Can you work these out from the model? Positions are in its coordinate system, mm. A direction names the side the tool comes from. Give positions to 0.01 mm unless a question says otherwise; leave off trailing zeros. Order: outer loops, then holes, each group sorted by start corner. A loop starts at its lowest first (then second) coordinate and runs counter-clockwise, first axis right, second up. Notation, with made-up numbers: (-4.5, 36) - (4.5, 36) arc R12 ccw to (4.5, 45) - close; hole circle Ø9 at (-12, 14.5). An arc over 180 degrees is marked (long way). Answer as a JSON object with one key per item and string values.
```python
from build123d import *

# Parameters (mm, degrees)
SKETCH1_W                                            = 160
SKETCH1_H                                            = 20
BOSS_EXTRUDE1_DEPTH                                  = 10
CBORE_FOR_M6_SLOTTED_CHEESE_HEAD_SCREWS2_D           = 6.6
CBORE_FOR_M6_SLOTTED_CHEESE_HEAD_SCREWS2_CBORE_D     = 11
CBORE_FOR_M6_SLOTTED_CHEESE_HEAD_SCREWS2_CBORE_DEPTH = 6.8
M6_TAPPED_HOLE1_D                                    = 5
M6_TAPPED_HOLE1_DEPTH                                = 15
M6_TAPPED_HOLE1_TIP                                  = 1.502151548
CHAMFER1_SIZE                                        = 5


with BuildPart() as part:
    # Sketch1 → Boss-Extrude1 (new, symmetric)
    with BuildSketch(Plane(origin=(0, 0, 0), x_dir=(1, 0, 0), z_dir=(0, 1, 0))):
        Rectangle(SKETCH1_W, SKETCH1_H)
    extrude(amount=BOSS_EXTRUDE1_DEPTH, both=True)

    # CBORE for M6 Slotted cheese head screws2 (through all)
    with Locations(Plane(origin=(0, 10, 0), x_dir=(1, 0, 0), z_dir=(0, 1, 0))):
        with Locations((-16.182, 0), (63.818, 0)):
            CounterBoreHole(CBORE_FOR_M6_SLOTTED_CHEESE_HEAD_SCREWS2_D / 2, CBORE_FOR_M6_SLOTTED_CHEESE_HEAD_SCREWS2_CBORE_D / 2, CBORE_FOR_M6_SLOTTED_CHEESE_HEAD_SCREWS2_CBORE_DEPTH)

    # M6 Tapped Hole1
    with Locations(Plane.ZY.offset(80)):
        with Locations((0, 0)):
            Hole(M6_TAPPED_HOLE1_D / 2, depth=M6_TAPPED_HOLE1_DEPTH)
            with Locations((0, 0, -(M6_TAPPED_HOLE1_DEPTH + M6_TAPPED_HOLE1_TIP / 2))):  # 118° drill point
                Cone(0, M6_TAPPED_HOLE1_D / 2, M6_TAPPED_HOLE1_TIP, mode=Mode.SUBTRACT)

    # Chamfer1
    chamfer1_edges = [part.edges().sort_by_distance(p)[0] for p in [
        (80, 10, 0),
    ]]
    chamfer(chamfer1_edges, length=CHAMFER1_SIZE)


solid = part.part
```
Q1. I'm going to push flat-ended pins straight in: pin 1 Ø6 at (x, z) = (-16.182, 0) entering from -Y; pin 2 Ø10.5 at (x, z) = (63.818, 0) entering from +Y. Where does each tip first touch, or does it pass through?
Recorded:
{"pin 1": "passes through", "pin 2": "stops at y = 3.2"}
Q2. I need wall thicknesses on L1, parallel to X at y = 9.25, z = 4.5; L2, parallel to X at y = 8.25, z = 4; L3, parallel to Y at x = -14.5, z = 4. Which ranges of each line are inside material? Lowest first, please.
Recorded:
{"L1": "x = -80 to -19.34, -13.02 to 60.66, 66.98 to 75.75", "L2": "x = -80 to -19.96, -12.41 to 60.04, 67.59 to 76.75", "L3": "y = -10 to 3.2"}
Q3. If we section it at A-A, the plane y = -6.5: Please give me the cut outline in (x, z), then the cut area to 3 significant figures.
Recorded:
{"outline": "(-80, -10) - (80, -10) - (80, 10) - (-80, 10) - close; hole circle Ø6.6 at (-16.18, 0); hole circle Ø6.6 at (63.82, 0)", "area": "3,130 mm^2"}
Q4. We'd pull the mould along X, two halves only. Please class faces 1 (the face through (64, 3.2, 4)), 2 (the face through (80, -2, 0)), 3 (the face through (-80, -2, 2)): released by +X, released by -X, zero draft, split by the parting line, or undercut.
Recorded:
{"face 1": "undercut", "face 2": "released by +X", "face 3": "released by -X"}
Q5. Which directions (+Z, -Z, +X, -X, +Y, -Y) give clear straight access to the entire face, cutting with the end or side of a thin tool? Please do faces 4 (the face through (-72.4, -2.44, 0.54)), 5 (the face through (-21.677, 6.648, -0.242)), 6 (the face through (-19.23, -3.49, 1.26)).
Recorded:
{"face 4": "-X", "face 5": "+Y", "face 6": "+Y, -Y"}
